Can you work these out from the model? Positions are in its coordinate system, mm. A direction names the side the tool comes from. Give positions to 0.01 mm unless a question says otherwise; leave off trailing zeros. Write each loop counter-clockwise with the first axis right and the second up, starting at its lowest first coordinate (ties: lowest second). Pieces come first, ordered by that corner, then holes. Notation, with made-up numbers: M -9,52 L 21,52 A13 cw 21,71 Z; hole C 67.25,38.25 d5. An arc over 180 degrees is marked long. Use CSV: the item, a comma, the result in double quotes. Start each with the question number.
Autodesk Inventor part; units mm, degrees
ref_plane "YZ Plane" through (0, 0, 0) normal (1, 0, 0) x (0, 1, 0)
ref_plane "XZ Plane" through (0, 0, 0) normal (0, 1, 0) x (-1, 0, 0)
ref_plane "XY Plane" through (0, 0, 0) normal (0, 0, 1) x (1, 0, 0)
sketch "Sketch1" plane through (0, 0, 0) normal (0, 1, 0) x (-1, 0, 0)
  line L0 (0, 0) -> (19.05, 0)
  line L1 (19.05, 0) -> (19.05, -19.05)
  line L2 (19.05, -19.05) -> (0, -19.05)
  line L3 (0, -19.05) -> (0, 0)
  line L4 (16.51, -16.51) -> (16.51, -2.54)
  line L5 (16.51, -2.54) -> (2.54, -2.54)
  line L6 (2.54, -2.54) -> (2.54, -16.51)
  line L7 (2.54, -16.51) -> (16.51, -16.51)
  dimension "d0" = 19.05
  dimension "d1" = 19.05
  dimension "d2" = 2.54
extrude "Extrusion1" add sketch "Sketch1" against normal blind 101.6
properties part number "Aluminum channel2"
(1) I want a section at A-A (x = -7). Write out the boundary of the cut face in (y, z).
(2) I want a section at C-C (y = -69.5). Write out the boundary of the cut face in (x, z), and give its area (3 significant figures).
(3) I want a section at B-B (z = -13). Write out the boundary of the cut face in (x, y), and give its area (3 significant figures).
(4) Please list where this line runs through material, in increasing order: L1, parallel to Z at x = -4.5, y = -18.5. Write a range as [from, to].
(5) Thinking about a two-plate mould opening in Z: for faces 3 (the face through (-2.54, -50, -9)), 4 (the face through (-19.05, -50, -9)), 5 (the face through (-10, -50, -19.05)), which applies, released by +Z, released by -Z, zero draft, split by the parting line, or undercut?
(6) Which directions (+Z, -Z, +X, -X, +Y, -Y) give clear straight access to the entire face, cutting with the end or side of a thin tool? Please do faces 1 (the face through (0, -50, -10)), 2 (the face through (-9, -50, -16.51)).
Geometry results:
1,outline,"M -101.6,-19.05 L 0,-19.05 L 0,-16.51 L -101.6,-16.51 Z; M -101.6,-2.54 L 0,-2.54 L 0,0 L -101.6,0 Z"
2,outline,"M -19.05,-19.05 L 0,-19.05 L 0,0 L -19.05,0 Z; hole M -16.51,-16.51 L -2.54,-16.51 L -2.54,-2.54 L -16.51,-2.54 Z"
2,area,"168 mm2"
3,outline,"M -19.05,-101.6 L -16.51,-101.6 L -16.51,0 L -19.05,0 Z; M -2.54,-101.6 L 0,-101.6 L 0,0 L -2.54,0 Z"
3,area,"516 mm2"
4,L1,"z = [-19.05, -16.51], [-2.54, 0]"
5,face 3,"undercut"
5,face 4,"zero draft"
5,face 5,"released by -Z"
6,face 1,"+Z, -Z, +X, +Y, -Y"
6,face 2,"+Y, -Y"
